from build123d import *

# Parameters (mm, degrees)
SKETCH_1_W          = 8
SKETCH_1_H          = 8
EXTRUDE_1_DEPTH     = 35
SKETCH_2_R          = 1.65
CUT_EXTRUDE_1_DEPTH = 40
SKETCH_3_R          = 1.65
CUT_EXTRUDE_2_DEPTH = 40


with BuildPart() as part:
    # 草图1 → 凸台-拉伸1 (new body)
    with BuildSketch(Plane.XY):
        with Locations((4, 4)):
            Rectangle(SKETCH_1_W, SKETCH_1_H)
    extrude(amount=EXTRUDE_1_DEPTH)

    # 草图2 → 切除-拉伸1 (cut)
    with BuildSketch(Plane(origin=(8, 0, 0), x_dir=(0, 0, -1), z_dir=(1, 0, 0))):
        with Locations(Location((-32.5, 4, 0), (0, 0, 90))):
            Circle(SKETCH_2_R)
        with Locations(Location((-2.5, 4, 0), (0, 0, 90))):
            Circle(SKETCH_2_R)
    extrude(amount=-CUT_EXTRUDE_1_DEPTH, mode=Mode.SUBTRACT)

    # 草图3 → 切除-拉伸2 (cut)
    with BuildSketch(Plane(origin=(0, 8, 0), x_dir=(1, 0, 0), z_dir=(0, 1, 0))):
        with Locations(Location((4, -17.5, 0), (0, 0, 270))):
            Circle(SKETCH_3_R)
    extrude(amount=-CUT_EXTRUDE_2_DEPTH, mode=Mode.SUBTRACT)


solid = part.part
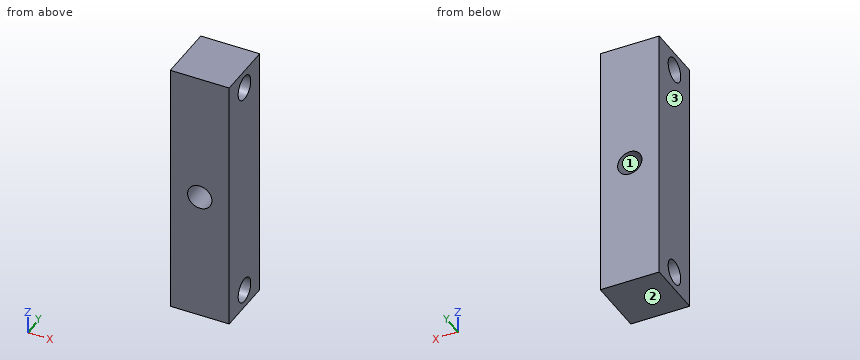
Could you check a few things on this model? Use its own coordinates, in mm. Face numbers are marked on the shaded views. Round coordinates to 2 decimals unless told otherwise and drop trailing zeros. Write each loop counter-clockwise with the first axis right and the second up, starting at its lowest first coordinate (ties: lowest second). Pieces come first, ordered by that corner, then holes. Notation, with made-up numbers: (24, 18) -> (55, 18) arc R26 ccw to (55, 38) -> close; hole circle Ø6 at (-5, 12). An arc over 180 degrees is marked (long way). Use a Markdown table: item, result.
1. If we section it at A-A (x = 4): List the corners of the cut face in (y, z) for me, then the cut area to 3 significant figures.
Answer key:
| item | result |
|---|---|
| outline | (0, 0) -> (8, 0) -> (8, 15.85) -> (0, 15.85) -> close; (0, 19.15) -> (8, 19.15) -> (8, 35) -> (0, 35) -> close; hole circle Ø3.3 at (4, 2.5); hole circle Ø3.3 at (4, 32.5) |
| area | 236 mm^2 |
2. If we section it at D-D (y = 7.5): List the corners of the cut face in (x, z) for me, then the cut area to 3 significant figures.
Answer key:
| item | result |
|---|---|
| outline | (0, 0) -> (8, 0) -> (8, 35) -> (0, 35) -> close; hole circle Ø3.3 at (4, 17.5) |
| area | 271 mm^2 |
3. If we section it at B-B (y = 4.25): List the corners of the cut face in (x, z) for me, then the cut area to 3 significant figures.
Answer key:
| item | result |
|---|---|
| outline | (0, 0) -> (8, 0) -> (8, 0.87) -> (0, 0.87) -> close; (0, 4.13) -> (8, 4.13) -> (8, 30.87) -> (0, 30.87) -> close; (0, 34.13) -> (8, 34.13) -> (8, 35) -> (0, 35) -> close; hole circle Ø3.3 at (4, 17.5) |
| area | 219 mm^2 |
4. For pin 1 Ø2.5 at (x, z) = (4, 17.5) entering from +Y, with a flat end and sliding along its axis, tell me the tip position at first contact or that it passes through.
Answer key:
| item | result |
|---|---|
| pin 1 | passes through |
5. We'd pull the mould along Z, two halves only. Please class the marked faces 1, 2 and 3: +Z half, -Z half, draft (parallel to the pull), parting line (faces both ways), or undercut.
Answer key:
| item | result |
|---|---|
| face 1 | undercut |
| face 2 | -Z half |
| face 3 | draft |
6. If we section it at C-C (z = 2.5): List the corners of the cut face in (x, y) for me.
Answer key:
| item | result |
|---|---|
| outline | (0, 0) -> (8, 0) -> (8, 2.35) -> (0, 2.35) -> close; (0, 5.65) -> (8, 5.65) -> (8, 8) -> (0, 8) -> close |
7. Please list where these lines run through material, in increasing order: probe 1 along Z at (x, y) = (5.75, 4); probe 2 along Z at (x, y) = (4.5, 4); probe 3 along Z at (x, y) = (4.75, 4).
Answer key:
| item | result |
|---|---|
| probe 1 | z = 0 to 0.85, 4.15 to 30.85, 34.15 to 35 |
| probe 2 | z = 0 to 0.85, 4.15 to 15.93, 19.07 to 30.85, 34.15 to 35 |
| probe 3 | z = 0 to 0.85, 4.15 to 16.03, 18.97 to 30.85, 34.15 to 35 |
